Autodesk Inventor part; units mm, degrees
ref_plane "YZ Plane" through (0, 0, 0) normal (1, 0, 0) x (0, 1, 0)
ref_plane "XZ Plane" through (0, 0, 0) normal (0, 1, 0) x (-1, 0, 0)
ref_plane "XY Plane" through (0, 0, 0) normal (0, 0, 1) x (1, 0, 0)
sketch "Skizze1" plane through (0, 0, 0) normal (1, 0, 0) x (0, 1, 0)
  line L0 (-8.5, -15) -> (8.5, -15)
  line L1 (8.5, -15) -> (8.5, 15)
  line L2 (8.5, 15) -> (-8.5, 15)
  line L3 (-8.5, 15) -> (-8.5, -15)
  line L4 (-8.5, -15) -> (8.5, 15) construction
  line L5 (8.5, -15) -> (-8.5, 15) construction
  line L6 (-8.5, -15) -> (21.5, -15)
  line L7 (21.5, -15) -> (8.5, 15)
  point P0 (0, 0)
  point P1 (8.5, -15)
  dimension "d0" = 30
  dimension "d1" = 17
  dimension "d3" = 30
extrude "Extrusion1" add sketch "Skizze1" along normal blind 30
sketch "Skizze2" plane through (0, -8.5, -15) normal (0, 0, -1) x (-1, 0, 0)
  line L0 (0, 30) -> (-30, 30) construction
  line L1 (-15, 30) -> (-15, 0) construction
  line L2 (0, 0) -> (-30, 0) construction
  line L3 (0, 17) -> (0, 0) construction
  line L4 (0, 15) -> (-30, 15) construction
  circle A0 centre (-15, 15) radius 2.15
  point P0 (0, 8.5)
  dimension "d6" = 4.3
extrude "Extrusion2" cut sketch "Skizze2" against normal blind 2
sketch "Skizze4" plane through (0, -8.5, -15) normal (0, -1, 0) x (1, 0, 0)
  line L0 (0, 30) -> (30, 30) construction
  line L1 (15, 30) -> (15, 0) construction
  line L2 (17.15, 0) -> (12.85, 0) construction
  line L3 (7.5, 4) -> (22.5, 4)
  line L4 (0, 0) -> (30, 0)
  line L5 (0, 30) -> (0, 0)
  line L6 (7.5, 4) -> (11.5, 0)
  line L7 (0, 0) -> (30, 0)
  line L8 (22.5, 4) -> (18.5, 0)
  line L9 (7.5, -4) -> (22.5, -4)
  line L10 (7.5, -4) -> (11.5, 0)
  line L11 (22.5, -4) -> (18.5, 0)
  point P0 (0, 15)
  dimension "d9" = 4
  dimension "d10" = 15
  dimension "d11" = 7.5
  dimension "d12" = 45
extrude "Extrusion3" add sketch "Skizze4" against normal blind 30 contours L4 L11 L9 L10
properties part number "CarlaRescueRampeTeil2"
Could you check a few things on this model? Use its own coordinates, in mm. A direction names the side the tool comes from. Give positions to 0.01 mm unless a question says otherwise; leave off trailing zeros. Loops run counter-clockwise (first coordinate to the right, second up) from the corner with the lowest first, then second, coordinate; pieces in that order, holes last. Notation, with made-up numbers: (18, -10.75) - (25, -10.75) arc R32 ccw to (25, 23.25) - close; hole circle Ø6 at (38.5, 30). An arc over 180 degrees is marked (long way). Use one line per item in the form item = value.
1. I want a section at B-B (y = 6.5). Please give me the cut outline in (x, z), and give its area (3 significant figures).
Response values:
outline = (0, -15) - (11.5, -15) - (7.5, -19) - (22.5, -19) - (18.5, -15) - (30, -15) - (30, 15) - (0, 15) - close; hole (12.85, -15) - (17.15, -15) - (17.15, -13) - (12.85, -13) - close
area = 935 mm²
2. I want a section at D-D (y = 0). Please give me the cut outline in (x, z), and give its area (3 significant figures).
Response values:
outline = (0, -15) - (11.5, -15) - (7.5, -19) - (22.5, -19) - (18.5, -15) - (30, -15) - (30, 15) - (0, 15) - close
area = 944 mm²
3. I need wall thicknesses on probe 1 along Z at (x, y) = (15, 15); probe 2 along Z at (x, y) = (24, 2.75); probe 3 along Y at (x, z) = (15, -14.35). Which ranges of each line are inside material? Lowest first, please.
Response values:
probe_1 = -19 to 0
probe_2 = -15 to 15
probe_3 = -8.5 to 4.35, 8.65 to 21.22
4. On a 3-axis mill with a long thin cutter (end or side, diameter ignored), from which of +Z, -Z, +X, -X, +Y, -Y can I reach the whole of each face in a straight line? I mean faces 1 (the face through (15, 6, -15)), 2 (the face through (24, 6, -15)), 3 (the face through (9.5, 6.3, -17)), 4 (the face through (15, 15, 0)), 5 (the face through (15, 6, -19)). Say none if no direction works.
Response values:
face_1 = none
face_2 = +X, +Y, -Y
face_3 = -X, +Y, -Y
face_4 = +Z, +X, -X, +Y
face_5 = -Z, +X, -X, +Y, -Y
5. I'm going to push a flat-ended pin straight in: pin 1 Ø1 at (x, y) = (20.5, 13.5) entering from +Z. Where does the tip first touch, or does it pass through?
Response values:
pin_1 = 4.62
6. Thinking about a two-plate mould opening in Y: for faces 6 (the face through (15, 7, -13)), 7 (the face through (15, -8.5, -2)), 8 (the face through (20.5, 6.3, -17)), which applies, released by +Y, released by -Y, zero draft, split by the parting line, or undercut?
Response values:
face_6 = undercut
face_7 = released by -Y
face_8 = zero draft
7. I want a section at C-C (x = 15). Please give me the cut outline in (y, z).
Response values:
outline = (-8.5, -19) - (21.5, -19) - (21.5, -15) - (8.5, 15) - (-8.5, 15) - close; hole (4.35, -15) - (8.65, -15) - (8.65, -13) - (4.35, -13) - close
8. I want a section at A-A (x = 11). Please give me the cut outline in (y, z), and give its area (3 significant figures).
Response values:
outline = (-8.5, -19) - (21.5, -19) - (21.5, -15.5) - (-8.5, -15.5) - close; (-8.5, -15) - (21.5, -15) - (8.5, 15) - (-8.5, 15) - close
area = 810 mm²
